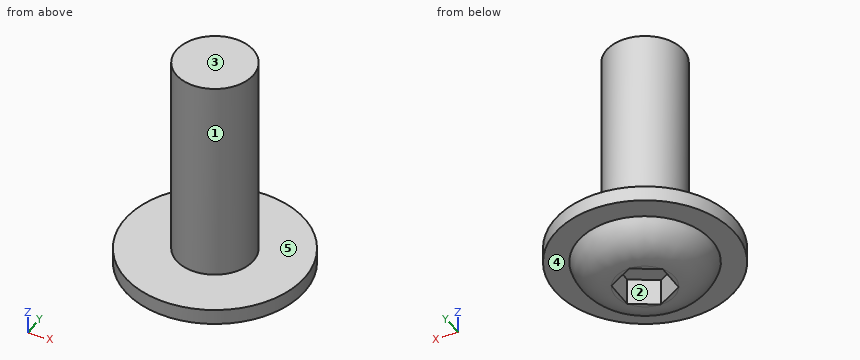
Autodesk Inventor part; units mm, degrees
ref_plane "YZ Plane" through (0, 0, 0) normal (1, 0, 0) x (0, 1, 0)
ref_plane "XZ Plane" through (0, 0, 0) normal (0, 1, 0) x (-1, 0, 0)
ref_plane "XY Plane" through (0, 0, 0) normal (0, 0, 1) x (1, 0, 0)
sketch "スケッチ1" plane through (0, 0, 0) normal (0, 1, 0) x (-1, 0, 0)
  line L0 (0, 0) -> (-1.1547, 0)
  line L1 (-2.6, 1.05) -> (-3.5, 1.05)
  line L2 (-3.5, 1.05) -> (-3.5, 1.65)
  line L3 (-3.5, 1.65) -> (-1.5, 1.65)
  line L4 (-1.5, 1.65) -> (-1.5, 9.65)
  line L5 (-1.5, 9.65) -> (0, 9.65)
  line L6 (0, 9.65) -> (0, 0)
  arc A0 (-2.6, 1.05) -> (-1.1547, 0) centre (-1.1547, 1.5197) ccw
  dimension "d0" = 5.2
  dimension "d1" = 7
  dimension "d3" = 1.65
  dimension "d4" = 0.6
  dimension "d5" = 2.3094
  dimension "d6" = 8
  dimension "d7" = 3
revolve "回転1" add sketch "スケッチ1" angle 360 about axis through (0, 0, 9.65) along (0, 0, -1)
thread "ねじ1"
sketch "スケッチ2" plane through (0, 0, 0) normal (0, 0, -1) x (-1, 0, 0)
  circle A0 centre (0, 0) radius 1.1547
  line L0 (0, 1.1547) -> (1, 0.5774)
  line L1 (1, 0.5774) -> (1, -0.5774)
  line L2 (1, -0.5774) -> (0, -1.1547)
  line L3 (0, -1.1547) -> (-1, -0.5774)
  line L4 (-1, -0.5774) -> (-1, 0.5774)
  line L5 (-1, 0.5774) -> (0, 1.1547)
  point P0 (0, 0)
extrude "押し出し1" cut sketch "スケッチ2" against normal blind 1.05 contours L1 L2 L3 L4 L5 L0
properties part number "620103008" material "ステンレス鋼 AISI 304"
Could you check a few things on this model? Use its own coordinates, in mm. Face numbers are marked on the shaded views. A direction names the side the tool comes from. Round coordinates to 2 decimals unless told otherwise and drop trailing zeros. Write each loop counter-clockwise with the first axis right and the second up, starting at its lowest first coordinate (ties: lowest second). Pieces come first, ordered by that corner, then holes. Notation, with made-up numbers: (79.25, -17.75) - (131.25, -17.75) arc R33 ccw to (131.25, 10.25) - close; hole circle Ø11 at (-11.75, -3.5). An arc over 180 degrees is marked (long way). Use a Markdown table: item, result.
Q1. Please list where these lines run through material, in increasing order: L1, parallel to X at y = 0, z = 9.25; L2, parallel to Z at x = -0.75, y = -1; L3, parallel to Z at x = 0.75, y = 0.
Output values:
| item | result |
|---|---|
| L1 | -1.5 to 1.5 |
| L2 | 0 to 9.65 |
| L3 | 1.05 to 9.65 |
Q2. For pin 1 (0.5 mm diameter, centred on y = 0, z = 0.5, fed in from +X); pin 2 (0.8 mm diameter, centred on y = 0, z = 0.5, fed in from -X); pin 3 (1.5 mm diameter, centred on x = 0.5, z = 4, fed in from -Y), each with a flat end and sliding along its axis, tell me the tip position at first contact or that it passes through.
Output values:
| item | result |
|---|---|
| pin 1 | x = 2.47 |
| pin 2 | x = -2.54 |
| pin 3 | y = -1.5 |
Q3. I want a section at B-B (y = 2.75). List the corners of the cut face in (x, z) for me, plus the area to 3 significant figures.
Output values:
| item | result |
|---|---|
| outline | (-2.17, 1.05) - (2.17, 1.05) - (2.17, 1.65) - (-2.17, 1.65) - close |
| area | 2.60 mm2 |
Q4. Thinking about a two-plate mould opening in X: for the marked faces 1, 2 and 3, which applies, released by +X, released by -X, zero draft, split by the parting line, or undercut?
Output values:
| item | result |
|---|---|
| face 1 | split by the parting line |
| face 2 | undercut |
| face 3 | zero draft |
Q5. I want a section at A-A (z = 7.25). List the corners of the cut face in (x, y) for me, plus the area to 3 significant figures.
Output values:
| item | result |
|---|---|
| outline | circle Ø3 at (0, 0) |
| area | 7.07 mm2 |
Q6. For the marked faces 4 and 5, which set-ups out of +Z, -Z, +X, -X, +Y, -Y let a thin tool reach every point of the face, with its end or its side?
Output values:
| item | result |
|---|---|
| face 4 | -Z |
| face 5 | +Z |
Q7. I want a section at C-C (z = 1.25). List the corners of the cut face in (x, y) for me.
Output values:
| item | result |
|---|---|
| outline | circle Ø7 at (0, 0) |
